Design review of the part built by this model. Coordinates are the model's own, in mm. Coordinates: 2 decimals unless noted, no trailing zeros. Write each loop counter-clockwise with the first axis right and the second up, starting at its lowest first coordinate (ties: lowest second). Pieces come first, ordered by that corner, then holes. Notation, with made-up numbers: (48.25, -2.5) - (79.25, -2.5) arc R23 cw to (79.25, 12.5) - close; hole circle Ø5 at (82.25, -29). An arc over 180 degrees is marked (long way). Answer as a JSON object with one key per item and string values.
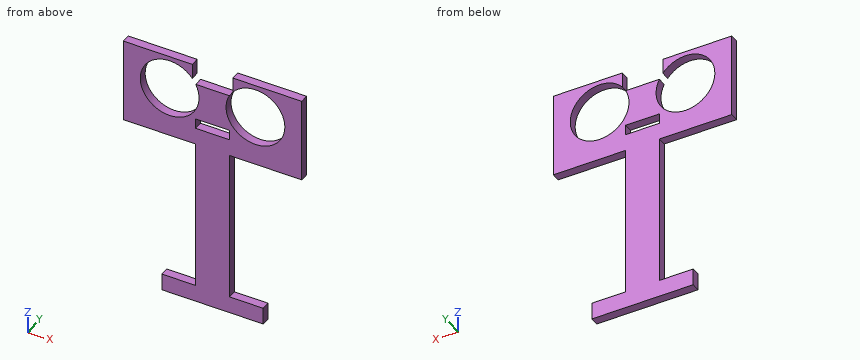
```python
from build123d import *

# Parameters (mm, degrees)
SKETCH1_W           = 10
SKETCH1_H           = 3
BOSS_EXTRUDE2_DEPTH = 2.54


with BuildPart() as part:
    # Sketch1 → Boss-Extrude2 (new body)
    with BuildSketch(Plane(origin=(0, 0, 0), x_dir=(1, 0, 0), z_dir=(0, 1, 0))):
        with BuildLine():
            Line((-12.751841201, 24.899770263), (-2.751841201, 24.899770263))
            Line((-2.751841201, 24.899770263), (-2.751841201, -20.100229737))
            Line((-2.751841201, -20.100229737), (-24.151841201, -20.100229737))
            Line((-24.151841201, -20.100229737), (-24.151841201, -45.100229737))
            Line((-24.151841201, -45.100229737), (-3.751841201, -45.100229737))
            Line((-3.751841201, -45.100229737), (-3.751841201, -40.650004508))
            ThreePointArc((-3.751841201, -40.650004508), (-17.706309974, -30.297867525), (-2.725910836, -39.100229737))
            Line((-2.725910836, -39.100229737), (7.222228435, -39.100229737))
            ThreePointArc((7.222228435, -39.100229737), (22.202627573, -30.297867525), (8.248158799, -40.650004508))
            Line((8.248158799, -40.650004508), (8.248158799, -45.100229737))
            Line((8.248158799, -45.100229737), (28.648158799, -45.100229737))
            Line((28.648158799, -45.100229737), (28.648158799, -20.100229737))
            Line((28.648158799, -20.100229737), (7.248158799, -20.100229737))
            Line((7.248158799, -20.100229737), (7.248158799, 24.899770263))
            Line((7.248158799, 24.899770263), (17.248158799, 24.899770263))
            Line((17.248158799, 24.899770263), (17.248158799, 29.899770263))
            Line((17.248158799, 29.899770263), (-12.751841201, 29.899770263))
            Line((-12.751841201, 29.899770263), (-12.751841201, 24.899770263))
        make_face()
        with Locations((2.248158799, -26.600229737)):
            Rectangle(SKETCH1_W, SKETCH1_H, mode=Mode.SUBTRACT)
    extrude(amount=BOSS_EXTRUDE2_DEPTH)


solid = part.part
```
(1) Take a section at C-C, the plane x = 11.5. Write out the cut boundary in (y, z), and give its area (3 significant figures).
Solved:
{"outline": "(0, -29.9) - (2.54, -29.9) - (2.54, -24.9) - (0, -24.9) - close; (0, 20.1) - (2.54, 20.1) - (2.54, 27.11) - (0, 27.11) - close; (0, 43.09) - (2.54, 43.09) - (2.54, 45.1) - (0, 45.1) - close", "area": "35.6 mm^2"}
(2) To check wall thickness, follow line 1 (Z direction, x = 14.5, y = 0.3); line 2 (Z direction, x = 8.5, y = 0.25); line 3 (Z direction, x = 6, y = 2.05). State the ranges of each line that lie inside material, in increasing order. Write a range as from..to.
Solved:
{"line 1": "z = -29.9..-24.9, 20.1..26.41, 43.79..45.1", "line 2": "z = -29.9..-24.9, 20.1..29.26, 40.94..45.1", "line 3": "z = -29.9..25.1, 28.1..39.1"}
(3) For pin 1 (0.8 mm diameter, centred on x = 3, y = 2, fed in from +Z); pin 2 (1 mm diameter, centred on y = 1, z = -9, fed in from +X); pin 3 (1.3 mm diameter, centred on y = 1, z = -27.5, fed in from +X), all flat-tipped, find the tip position at first contact; note any pin that passes through.
Solved:
{"pin 1": "stops at z = 39.1", "pin 2": "stops at x = 7.25", "pin 3": "stops at x = 17.25"}
(4) Take a section at D-D, the plane z = -12. Write out the cut boundary in (x, y), and give its area (3 significant figures).
Solved:
{"outline": "(-2.75, 0) - (7.25, 0) - (7.25, 2.54) - (-2.75, 2.54) - close", "area": "25.4 mm^2"}
(5) Take a section at B-B, the plane x = -18. Write out the cut boundary in (y, z).
Solved:
{"outline": "(0, 20.1) - (2.54, 20.1) - (2.54, 30.77) - (0, 30.77) - close; (0, 39.43) - (2.54, 39.43) - (2.54, 45.1) - (0, 45.1) - close"}
(6) Take a section at A-A, the plane y = 0.5. Write out the cut boundary in (x, z), and give its area (3 significant figures).
Solved:
{"outline": "(-24.15, 20.1) - (-2.75, 20.1) - (-2.75, -24.9) - (-12.75, -24.9) - (-12.75, -29.9) - (17.25, -29.9) - (17.25, -24.9) - (7.25, -24.9) - (7.25, 20.1) - (28.65, 20.1) - (28.65, 45.1) - (8.25, 45.1) - (8.25, 40.65) arc R8.7 cw (long way) to (7.22, 39.1) - (-2.73, 39.1) arc R8.7 cw (long way) to (-3.75, 40.65) - (-3.75, 45.1) - (-24.15, 45.1) - close; hole (-2.75, 25.1) - (7.25, 25.1) - (7.25, 28.1) - (-2.75, 28.1) - close", "area": "1,340 mm^2"}
